```python
from build123d import *

# Parameters (mm, degrees)
F0_W     = 50.8
F0_H     = 50.8
F0_R     = 12.7
F1_DEPTH = 50.8
F3_D     = 25.4
F5_D     = 25.4


# Not quite as in the source:
# - the program builds the solid bodies; features that only make, move or delete a surface that nothing else refers to are left out


with BuildPart() as f1:
    # F0 (on Right) → F1 (new body)
    with BuildSketch(Plane.YZ):
        Rectangle(F0_W, F0_H)
        Circle(F0_R, mode=Mode.SUBTRACT)
        Circle(F0_R)
    extrude(amount=F1_DEPTH)

    # F3 (through all)
    with Locations(Plane(origin=(0, 25.4, 0), x_dir=(-1, 0, 0), z_dir=(0, 1, 0))):
        with Locations((-25.4, 0)):
            Hole(F3_D / 2)

    # F5 (through all)
    with Locations(Plane.XY.offset(25.4)):
        with Locations((25.4, 0)):
            Hole(F5_D / 2)


solid = f1.part
```
Model file for the job. Use its own axes, mm. Give positions to 0.01 mm unless a question says otherwise; leave off trailing zeros. Write each loop counter-clockwise with the first axis right and the second up, starting at its lowest first coordinate (ties: lowest second). Pieces come first, ordered by that corner, then holes. Notation, with made-up numbers: M 77,14.25 L 126,14.25 A25 cw 126,44.25 Z; hole C 45.25,9.25 d4. An arc over 180 degrees is marked long. Use a Markdown table: item, result.
1) Drill centre lines: line 1 (X direction, y = 0, z = 6); line 2 (Y direction, x = 25, z = 15); line 3 (Z direction, x = 25.4, y = 14). Where is each one in solid material? Low to high. Write a range as from..to.
Responses:
| item | result |
|---|---|
| line 1 | x = 0..12.7, 38.1..50.8 |
| line 2 | y = -25.4..-12.69, 12.69..25.4 |
| line 3 | z = -25.4..-12.7, 12.7..25.4 |
2) Cut at C-C (z = 18). List the corners of the cut face in (x, y).
Responses:
| item | result |
|---|---|
| outline | M 0,-25.4 L 50.8,-25.4 L 50.8,25.4 L 0,25.4 Z; hole C 25.4,0 d25.4 |
3) Cut at B-B (z = 11). List the corners of the cut face in (x, y).
Responses:
| item | result |
|---|---|
| outline | M 0,-25.4 L 19.05,-25.4 L 19.05,-11 A12.7 cw 19.05,11 L 19.05,25.4 L 0,25.4 Z; M 31.75,-25.4 L 50.8,-25.4 L 50.8,25.4 L 31.75,25.4 L 31.75,11 A12.7 cw 31.75,-11 Z |
4) Cut at D-D (y = -2). List the corners of the cut face in (x, z), and give its area (3 significant figures).
Responses:
| item | result |
|---|---|
| outline | M 0,-25.4 L 12.86,-25.4 L 12.86,-2 A12.7 cw 12.86,2 L 12.86,25.4 L 0,25.4 Z; M 37.94,-25.4 L 50.8,-25.4 L 50.8,25.4 L 37.94,25.4 L 37.94,2 A12.7 cw 37.94,-2 Z |
| area | 1,310 mm2 |
5) Pull direction Y, two halves, no side cores. Call faces 1 (the flat face through (14, 25.4, -6)), 2 (the cylindrical face through (35.5, -7.7, 15.3)), 3 (the flat face through (50.8, 0, 0)): +Y half, -Y half, draft (parallel to the pull), parting line (faces both ways), or undercut.
Responses:
| item | result |
|---|---|
| face 1 | +Y half |
| face 2 | undercut |
| face 3 | draft |
6) Cut at A-A (x = 25.4). List the corners of the cut face in (y, z).
Responses:
| item | result |
|---|---|
| outline | M -25.4,-25.4 L -12.7,-25.4 L -12.7,-12.7 L -25.4,-12.7 Z; M -25.4,12.7 L -12.7,12.7 L -12.7,25.4 L -25.4,25.4 Z; M 12.7,-25.4 L 25.4,-25.4 L 25.4,-12.7 L 12.7,-12.7 Z; M 12.7,12.7 L 25.4,12.7 L 25.4,25.4 L 12.7,25.4 Z |
